Part model, mm, in its own coordinate system. Round coordinates to 2 decimals unless told otherwise and drop trailing zeros. Write each loop counter-clockwise with the first axis right and the second up, starting at its lowest first coordinate (ties: lowest second). Pieces come first, ordered by that corner, then holes. Notation, with made-up numbers: M 12,2.25 L 40,2.25 A31 ccw 40,33.25 Z; hole C -25.75,26 d4. An arc over 180 degrees is marked long. One line per question, with ' | ' between items. Start each with the question number.
1) Saw through at B-B (x = -13). List the corners of the cut face in (y, z), plus the area to 3 significant figures.
2) Wall check: probe 1 along Z at (x, y) = (126, 5.75); probe 2 along Z at (x, y) = (-56.5, 7.25); probe 3 along X at (y, z) = (7, -254). Give the ranges that are in metal, low to high. Write a range as [from, to].
3) Saw through at D-D (z = -283). List the corners of the cut face in (x, y).
4) Mould opens along X. For faces 1 (the face through (-261.223, 4.93, -153.764)), 2 (the face through (-5, 10, -154)), 3 (the face through (79.969, 5.07, -195.318)) say: pulls with the +X half, pulls with the -X half, needs draft (parallel to the pull), parting line crosses it, or undercut.
5) Saw through at C-C (x = -164.5). List the corners of the cut face in (y, z).
6) Drop flat-ended pins along their axis: pin 1 Ø3 at (x, y) = (-88.5, 3.5) entering from +Z; pin 2 Ø4 at (x, z) = (-136.5, -159.5) entering from -Y; pin 3 Ø3 at (x, y) = (-205.5, 7.5) entering from -Z; pin 4 Ø5 at (y, z) = (4, -110.5) entering from +X. Give the stop position or say it passes through.
7) Saw through at A-A (z = -25). List the corners of the cut face in (x, y) (3 decimals), plus the area to 3 significant figures.
```python
from build123d import *

# Parameters (mm, degrees)
BOSS_EXTRUDE1_DEPTH = 10
SKETCH3_R           = 48.5
SKETCH3_R_2         = 50
SKETCH3_W           = 400
SKETCH3_H           = 65
CUT_EXTRUDE3_DEPTH  = 10
CUT_EXTRUDE4_DEPTH  = 10


with BuildPart() as part:
    # Sketch1 → Boss-Extrude1 (new body)
    with BuildSketch(Plane(origin=(0, 0, 0), x_dir=(1, 0, 0), z_dir=(0, 1, 0))):
        Polygon((175.101753381, 303.050121206), (-174.898226894, 303.167627278), (-349.999980275, 0.117506072), (-175.101753381, -303.050121206), (174.898226894, -303.167627278), (349.999980275, -0.117506072), align=None)
    extrude(amount=BOSS_EXTRUDE1_DEPTH)

    # Sketch3 → Cut-Extrude3 (cut)
    with BuildSketch(Plane(origin=(0, 10, 0), x_dir=(1, 0, 0), z_dir=(0, 1, 0))):
        with Locations(Location((249.999980275, 0, 0), (0, 0, 270))):
            Circle(SKETCH3_R)
        with Locations(Location((-250.000009417, 0.041161845, 0), (0, 0, 270))):
            Circle(SKETCH3_R_2)
        with Locations(Location((-126.076603066, 215.895357646, 0), (0, 0, 270))):
            Circle(SKETCH3_R_2)
        with Locations(Location((122.996764387, 217.697498973, 0), (0, 0, 270))):
            Circle(SKETCH3_R)
        with Locations((0, 98.413699872)):
            Rectangle(SKETCH3_W, SKETCH3_H)
    extrude(amount=-CUT_EXTRUDE3_DEPTH, mode=Mode.SUBTRACT)

    # Sketch2 → Cut-Extrude4 (cut)
    with BuildSketch(Plane(origin=(0, 10, 0), x_dir=(1, 0, 0), z_dir=(0, 1, 0))):
        Polygon((-175.101753381, -303.050121206), (174.898226894, -303.167627278), (349.999980275, -0.117506072), (-349.999980275, 0.117506072), align=None)
    extrude(amount=-CUT_EXTRUDE4_DEPTH, mode=Mode.SUBTRACT)


solid = part.part
```
Answer key:
1) outline: M 0,-303.11 L 10,-303.11 L 10,-130.91 L 0,-130.91 Z; M 0,-65.91 L 10,-65.91 L 10,0 L 0,0 Z | area: 2,380 mm2
2) probe 1: z = [-303.07, -266.1], [-169.29, -130.91], [-65.91, 0.04] | probe 2: z = [-303.13, -130.91], [-65.91, -0.02] | probe 3: x = [-203.31, -158.45], [-93.7, 90.84], [155.16, 203.4]
3) outline: M -186.55,0 L 186.67,0 L 186.67,10 L -186.55,10 Z
4) face 1: pulls with the -X half | face 2: needs draft | face 3: undercut
5) outline: M 0,-303.16 L 10,-303.16 L 10,-247.89 L 0,-247.89 Z; M 0,-183.9 L 10,-183.9 L 10,-130.91 L 0,-130.91 Z; M 0,-65.91 L 10,-65.91 L 10,-0.06 L 0,-0.06 Z
6) pin 1: stops at z = -0.03 | pin 2: stops at y = 0 | pin 3: stops at z = -252.8 | pin 4: stops at x = 287.63
7) outline: M -335.623,0 L -293.325,0 L -293.325,10 L -335.623,10 Z; M -206.675,0 L 208.44,0 L 208.44,10 L -206.675,10 Z; M 291.56,0 L 335.51,0 L 335.51,10 L 291.56,10 Z | area: 5,010 mm2
